from build123d import *
from OCP.BRepFilletAPI import BRepFilletAPI_MakeChamfer

# Parameters (mm, degrees)
SKETCH1_W           = 16
SKETCH1_H           = 16
SKETCH1_R           = 5
BOSS_EXTRUDE1_DEPTH = 40
FILLET1_R           = 4.5
CUT_EXTRUDE1_START  = -5
CUT_EXTRUDE1_DEPTH  = 5
CHAMFER1_SIZE       = 0.8
CHAMFER1_SIZE2      = 0.461880215
CHAMFER2_SIZE       = 0.8
CHAMFER2_SIZE2      = 0.461880215
SKETCH3_R           = 5
SKETCH3_R_2         = 4.5
BOSS_EXTRUDE2_DEPTH = 15
SKETCH4_R           = 7.25
CUT_EXTRUDE2_DEPTH  = 2


with BuildPart() as part:
    # Sketch1 → Boss-Extrude1 (new body)
    with BuildSketch(Plane(origin=(0, 0, 0), x_dir=(1, 0, 0), z_dir=(0, 1, 0))):
        Rectangle(SKETCH1_W, SKETCH1_H)
        with Locations(Location((0, 0, 0), (0, 0, 270))):
            Circle(SKETCH1_R, mode=Mode.SUBTRACT)
    extrude(amount=BOSS_EXTRUDE1_DEPTH)

    # Fillet1
    fillet1_edges = [part.edges().sort_by_distance(p)[0] for p in [
        (8, 20, 8),
        (-8, 20, 8),
        (-8, 20, -8),
        (8, 20, -8),
    ]]
    fillet(fillet1_edges, radius=FILLET1_R)

    # Sketch2 → Cut-Extrude1 (cut)
    with BuildSketch(Plane(origin=(0, 40, 0), x_dir=(1, 0, 0), z_dir=(0, 1, 0)).offset(CUT_EXTRUDE1_START)):
        with BuildLine():
            ThreePointArc((5, 0), (4.985837438, -0.376065209), (4.943429983, -0.75))
            Line((4.943429983, -0.75), (8, -0.75))
            Line((8, -0.75), (8, 0.75))
            Line((8, 0.75), (4.943429983, 0.75))
            ThreePointArc((4.943429983, 0.75), (4.985837438, 0.376065209), (5, 0))
        make_face()
        with BuildLine():
            Line((-0.904749438, 8), (-0.904749438, 4.917461586))
            ThreePointArc((-0.904749438, 4.917461586), (0, 5), (0.904749438, 4.917461586))
            Line((0.904749438, 4.917461586), (0.904749438, 8))
            Line((0.904749438, 8), (-0.904749438, 8))
        make_face()
        with BuildLine():
            ThreePointArc((0.904749438, -4.917461586), (0, -5), (-0.904749438, -4.917461586))
            Line((-0.904749438, -4.917461586), (-0.904749438, -8))
            Line((-0.904749438, -8), (0.904749438, -8))
            Line((0.904749438, -8), (0.904749438, -4.917461586))
        make_face()
        with BuildLine():
            Line((-8, 0.75), (-8, -0.75))
            Line((-8, -0.75), (-4.943429983, -0.75))
            ThreePointArc((-4.943429983, -0.75), (-5, 0), (-4.943429983, 0.75))
            Line((-4.943429983, 0.75), (-8, 0.75))
        make_face()
    extrude(amount=CUT_EXTRUDE1_DEPTH, mode=Mode.SUBTRACT)

    # Chamfer1: one chamfer whose edges measure the first distance from different faces: ONE call of the kernel's chamfer builder (chamfer() names one face for all edges)
    chamfer1_edges_1 = [part.edges().sort_by_distance(p)[0] for p in [
        (6.471714992, 40, -0.75),
    ]]
    chamfer1_side_1 = [part.faces().sort_by_distance(p)[0] for p in [
        (6.471714992, 37.5, -0.75),
    ]]
    chamfer1_edges_2 = [part.edges().sort_by_distance(p)[0] for p in [
        (6.471714992, 40, 0.75),
    ]]
    chamfer1_side_2 = [part.faces().sort_by_distance(p)[0] for p in [
        (4.797663916, 40, 4.721192893),
    ]]
    chamfer1_edges_3 = [part.edges().sort_by_distance(p)[0] for p in [
        (0.904749438, 40, -6.458730793),
    ]]
    chamfer1_side_3 = [part.faces().sort_by_distance(p)[0] for p in [
        (0.904749438, 37.5, -6.458730793),
    ]]
    chamfer1_edges_4 = [part.edges().sort_by_distance(p)[0] for p in [
        (-0.904749438, 40, -6.458730793),
    ]]
    chamfer1_side_4 = [part.faces().sort_by_distance(p)[0] for p in [
        (-4.797663916, 40, -4.721192893),
    ]]
    chamfer1_edges_5 = [part.edges().sort_by_distance(p)[0] for p in [
        (0.904749438, 40, 6.458730793),
    ]]
    chamfer1_side_5 = [part.faces().sort_by_distance(p)[0] for p in [
        (0.904749438, 37.5, 6.458730793),
    ]]
    chamfer1_edges_6 = [part.edges().sort_by_distance(p)[0] for p in [
        (-0.904749438, 40, 6.458730793),
        (-6.471714992, 40, 0.75),
    ]]
    chamfer1_side_6 = [part.faces().sort_by_distance(p)[0] for p in [
        (-4.797663916, 40, 4.721192893),
    ]]
    chamfer1_edges_7 = [part.edges().sort_by_distance(p)[0] for p in [
        (-6.471714992, 40, -0.75),
    ]]
    chamfer1_side_7 = [part.faces().sort_by_distance(p)[0] for p in [
        (-6.471714992, 37.5, -0.75),
    ]]
    chamfer1 = BRepFilletAPI_MakeChamfer(part.part.solid().wrapped)
    for e in chamfer1_edges_1:
        chamfer1.Add(CHAMFER1_SIZE, CHAMFER1_SIZE2, e.wrapped, chamfer1_side_1[0].wrapped)  # the first distance lies on this face
    for e in chamfer1_edges_2:
        chamfer1.Add(CHAMFER1_SIZE, CHAMFER1_SIZE2, e.wrapped, chamfer1_side_2[0].wrapped)  # the first distance lies on this face
    for e in chamfer1_edges_3:
        chamfer1.Add(CHAMFER1_SIZE, CHAMFER1_SIZE2, e.wrapped, chamfer1_side_3[0].wrapped)  # the first distance lies on this face
    for e in chamfer1_edges_4:
        chamfer1.Add(CHAMFER1_SIZE, CHAMFER1_SIZE2, e.wrapped, chamfer1_side_4[0].wrapped)  # the first distance lies on this face
    for e in chamfer1_edges_5:
        chamfer1.Add(CHAMFER1_SIZE, CHAMFER1_SIZE2, e.wrapped, chamfer1_side_5[0].wrapped)  # the first distance lies on this face
    for e in chamfer1_edges_6:
        chamfer1.Add(CHAMFER1_SIZE, CHAMFER1_SIZE2, e.wrapped, chamfer1_side_6[0].wrapped)  # the first distance lies on this face
    for e in chamfer1_edges_7:
        chamfer1.Add(CHAMFER1_SIZE, CHAMFER1_SIZE2, e.wrapped, chamfer1_side_7[0].wrapped)  # the first distance lies on this face
    add(Compound.cast(chamfer1.Shape()), mode=Mode.REPLACE)

    # Chamfer2: one chamfer whose edges measure the first distance from different faces: ONE call of the kernel's chamfer builder (chamfer() names one face for all edges)
    chamfer2_edges_1 = [part.edges().sort_by_distance(p)[0] for p in [
        (-3.592924063, 40, 3.477196669),
    ]]
    chamfer2_side_1 = [part.faces().sort_by_distance(p)[0] for p in [
        (-4.956967709, 40, 4.876915228),
    ]]
    chamfer2_edges_2 = [part.edges().sort_by_distance(p)[0] for p in [
        (3.467104871, 40, 3.602663433),
    ]]
    chamfer2_side_2 = [part.faces().sort_by_distance(p)[0] for p in [
        (4.836216734, 40, 4.929925488),
    ]]
    chamfer2_edges_3 = [part.edges().sort_by_distance(p)[0] for p in [
        (3.59170795, 40, -3.478452817),
    ]]
    chamfer2_side_3 = [part.faces().sort_by_distance(p)[0] for p in [
        (4.888861893, 40, -4.810636969),
    ]]
    chamfer2_edges_4 = [part.edges().sort_by_distance(p)[0] for p in [
        (-3.713035057, 40, -3.348637136),
    ]]
    chamfer2_side_4 = [part.faces().sort_by_distance(p)[0] for p in [
        (-5.007269345, 40, -4.755258355),
    ]]
    chamfer2_edges_5 = [part.edges().sort_by_distance(p)[0] for p in [
        (-2.602374719, 40, -8),
        (2.433314827, 40, -8),
    ]]
    chamfer2_side_5 = [part.faces().sort_by_distance(p)[0] for p in [
        (7.6955e-05, 19.387827312, -8),
    ]]
    chamfer2_edges_6 = [part.edges().sort_by_distance(p)[0] for p in [
        (-8, 40, -2.355940108),
        (-8, 40, 2.525),
    ]]
    chamfer2_side_6 = [part.faces().sort_by_distance(p)[0] for p in [
        (-8, 19.4908238, -7.6518e-05),
    ]]
    chamfer2_edges_7 = [part.edges().sort_by_distance(p)[0] for p in [
        (-6.681980515, 40, -6.681980515),
    ]]
    chamfer2_side_7 = [part.faces().sort_by_distance(p)[0] for p in [
        (-6.681980515, 20, -6.681980515),
    ]]
    chamfer2_edges_8 = [part.edges().sort_by_distance(p)[0] for p in [
        (-2.602374719, 40, 8),
        (2.433314827, 40, 8),
    ]]
    chamfer2_side_8 = [part.faces().sort_by_distance(p)[0] for p in [
        (7.6955e-05, 19.387827312, 8),
    ]]
    chamfer2_edges_9 = [part.edges().sort_by_distance(p)[0] for p in [
        (-6.681980515, 40, 6.681980515),
    ]]
    chamfer2_side_9 = [part.faces().sort_by_distance(p)[0] for p in [
        (-6.681980515, 20, 6.681980515),
    ]]
    chamfer2_edges_10 = [part.edges().sort_by_distance(p)[0] for p in [
        (8, 40, 2.525),
        (8, 40, -2.355940108),
    ]]
    chamfer2_side_10 = [part.faces().sort_by_distance(p)[0] for p in [
        (8, 19.4908238, -7.6518e-05),
    ]]
    chamfer2_edges_11 = [part.edges().sort_by_distance(p)[0] for p in [
        (6.681980515, 40, 6.681980515),
    ]]
    chamfer2_side_11 = [part.faces().sort_by_distance(p)[0] for p in [
        (6.681980515, 20, 6.681980515),
    ]]
    chamfer2_edges_12 = [part.edges().sort_by_distance(p)[0] for p in [
        (6.681980515, 40, -6.681980515),
    ]]
    chamfer2_side_12 = [part.faces().sort_by_distance(p)[0] for p in [
        (6.681980515, 20, -6.681980515),
    ]]
    chamfer2 = BRepFilletAPI_MakeChamfer(part.part.solid().wrapped)
    for e in chamfer2_edges_1:
        chamfer2.Add(CHAMFER2_SIZE, CHAMFER2_SIZE2, e.wrapped, chamfer2_side_1[0].wrapped)  # the first distance lies on this face
    for e in chamfer2_edges_2:
        chamfer2.Add(CHAMFER2_SIZE, CHAMFER2_SIZE2, e.wrapped, chamfer2_side_2[0].wrapped)  # the first distance lies on this face
    for e in chamfer2_edges_3:
        chamfer2.Add(CHAMFER2_SIZE, CHAMFER2_SIZE2, e.wrapped, chamfer2_side_3[0].wrapped)  # the first distance lies on this face
    for e in chamfer2_edges_4:
        chamfer2.Add(CHAMFER2_SIZE, CHAMFER2_SIZE2, e.wrapped, chamfer2_side_4[0].wrapped)  # the first distance lies on this face
    for e in chamfer2_edges_5:
        chamfer2.Add(CHAMFER2_SIZE, CHAMFER2_SIZE2, e.wrapped, chamfer2_side_5[0].wrapped)  # the first distance lies on this face
    for e in chamfer2_edges_6:
        chamfer2.Add(CHAMFER2_SIZE, CHAMFER2_SIZE2, e.wrapped, chamfer2_side_6[0].wrapped)  # the first distance lies on this face
    for e in chamfer2_edges_7:
        chamfer2.Add(CHAMFER2_SIZE, CHAMFER2_SIZE2, e.wrapped, chamfer2_side_7[0].wrapped)  # the first distance lies on this face
    for e in chamfer2_edges_8:
        chamfer2.Add(CHAMFER2_SIZE, CHAMFER2_SIZE2, e.wrapped, chamfer2_side_8[0].wrapped)  # the first distance lies on this face
    for e in chamfer2_edges_9:
        chamfer2.Add(CHAMFER2_SIZE, CHAMFER2_SIZE2, e.wrapped, chamfer2_side_9[0].wrapped)  # the first distance lies on this face
    for e in chamfer2_edges_10:
        chamfer2.Add(CHAMFER2_SIZE, CHAMFER2_SIZE2, e.wrapped, chamfer2_side_10[0].wrapped)  # the first distance lies on this face
    for e in chamfer2_edges_11:
        chamfer2.Add(CHAMFER2_SIZE, CHAMFER2_SIZE2, e.wrapped, chamfer2_side_11[0].wrapped)  # the first distance lies on this face
    for e in chamfer2_edges_12:
        chamfer2.Add(CHAMFER2_SIZE, CHAMFER2_SIZE2, e.wrapped, chamfer2_side_12[0].wrapped)  # the first distance lies on this face
    add(Compound.cast(chamfer2.Shape()), mode=Mode.REPLACE)

    # Sketch3 → Boss-Extrude2 (add)
    with BuildSketch(Plane.XZ):
        with Locations(Location((0, 0, 0), (0, 0, 270))):
            Circle(SKETCH3_R)
        with Locations(Location((0, 0, 0), (0, 0, 270))):
            Circle(SKETCH3_R_2, mode=Mode.SUBTRACT)
    extrude(amount=-BOSS_EXTRUDE2_DEPTH)

    # Sketch4 → Cut-Extrude2 (cut)
    with BuildSketch(Plane.XZ):
        with Locations(Location((0, 0, 0), (0, 0, 270))):
            Circle(SKETCH4_R)
    extrude(amount=-CUT_EXTRUDE2_DEPTH, mode=Mode.SUBTRACT)


solid = part.part
CAD build for the part. Positions are in the model's coordinates, mm. A direction names the side the tool comes from. Give positions to 0.01 mm unless a question says otherwise; leave off trailing zeros. Order: outer loops, then holes, each group sorted by start corner. A loop starts at its lowest first (then second) coordinate and runs counter-clockwise, first axis right, second up. Notation, with made-up numbers: (25, 9) - (67, 9) arc R34 ccw to (67, 46) - close; hole circle Ø2 at (50, -21.75). An arc over 180 degrees is marked (long way). Answer in a Markdown table with one row per item.
1. Saw through at C-C, the plane z = 0. Give the cut face in (x, y).
Data:
| item | result |
|---|---|
| outline | (-8, 0) - (-7.25, 0) - (-7.25, 2) - (-4.5, 2) - (-4.5, 15) - (-5, 15) - (-5, 35) - (-8, 35) - close; (4.5, 2) - (7.25, 2) - (7.25, 0) - (8, 0) - (8, 35) - (5, 35) - (5, 15) - (4.5, 15) - close |
2. Tool access for faces 1 (the cylindrical face through (-2.777, 0.986, -6.697)), 2 (the flat face through (-6.394, 39.766, 1.144)), 3 (the flat face through (-1.299, 39.766, -6.381)): list every direction of +Z, -Z, +X, -X, +Y, -Y with a clear straight run to the whole face (end or side of a thin tool).
Data:
| item | result |
|---|---|
| face 1 | -Y |
| face 2 | +X, -X, +Y |
| face 3 | +Z, -Z, +Y |
3. Saw through at A-A, the plane x = 0. Give the cut face in (y, z).
Data:
| item | result |
|---|---|
| outline | (0, -8) - (35, -8) - (35, -5) - (15, -5) - (15, -4.5) - (2, -4.5) - (2, -7.25) - (0, -7.25) - close; (0, 7.25) - (2, 7.25) - (2, 4.5) - (15, 4.5) - (15, 5) - (35, 5) - (35, 8) - (0, 8) - close |
4. Flat gauge pins, fed straight in: pin 1 (2 mm diameter, centred on x = -0.5, z = -7, fed in from +Y); pin 2 (1.5 mm diameter, centred on x = -4.5, y = 13, fed in from +Z); pin 3 (0.8 mm diameter, centred on x = -6, z = 0.5, fed in from +Y); pin 4 (5 mm diameter, centred on y = 18, z = -6, fed in from +X). Where does each tip first touch, or does it go through?
Data:
| item | result |
|---|---|
| pin 1 | stops at y = 39.88 |
| pin 2 | stops at z = 7.99 |
| pin 3 | stops at y = 39.62 |
| pin 4 | stops at x = 8 |
5. Saw through at D-D, the plane y = 5. Give the cut face in (x, z).
Data:
| item | result |
|---|---|
| outline | (-8, -3.5) arc R4.5 ccw to (-3.5, -8) - (3.5, -8) arc R4.5 ccw to (8, -3.5) - (8, 3.5) arc R4.5 ccw to (3.5, 8) - (-3.5, 8) arc R4.5 ccw to (-8, 3.5) - close; hole circle Ø9 at (0, 0) |
6. Probe probe 1 along Z at (x, y) = (0, 23.5); probe 2 along X at (y, z) = (9.5, 0); probe 3 along X at (y, z) = (1.15, 0). List the from-to ranges inside material, lowest first. Write a range as [from, to].
Data:
| item | result |
|---|---|
| probe 1 | z = [-8, -5], [5, 8] |
| probe 2 | x = [-8, -4.5], [4.5, 8] |
| probe 3 | x = [-8, -7.25], [7.25, 8] |
7. Saw through at B-B, the plane y = 30. Give the cut face in (x, z).
Data:
| item | result |
|---|---|
| outline | (-8, -3.5) arc R4.5 ccw to (-3.5, -8) - (3.5, -8) arc R4.5 ccw to (8, -3.5) - (8, 3.5) arc R4.5 ccw to (3.5, 8) - (-3.5, 8) arc R4.5 ccw to (-8, 3.5) - close; hole circle Ø10 at (0, 0) |
8. Pull direction Z, two halves, no side cores. Call faces 4 (the flat face through (-5, 2, 0)), 5 (the flat face through (-0.905, 37, 6)), 6 (the flat face through (0, 19, -8)): pulls with the +Z half, pulls with the -Z half, needs draft (parallel to the pull), parting line crosses it, or undercut.
Data:
| item | result |
|---|---|
| face 4 | undercut |
| face 5 | needs draft |
| face 6 | pulls with the -Z half |
